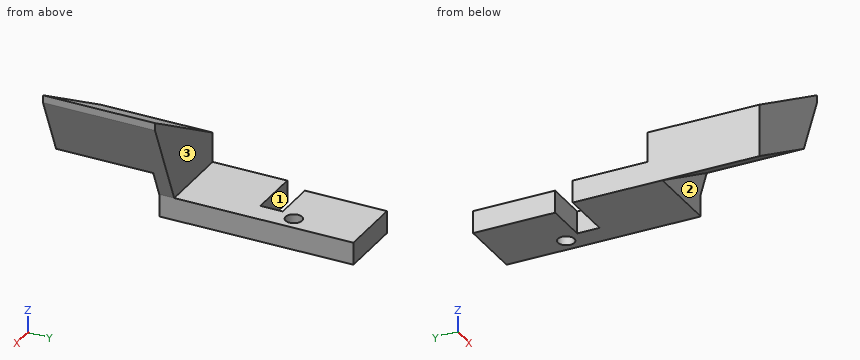
from build123d import *

# Parameters (mm, degrees)
SKETCH1_R           = 1.1
BOSS_EXTRUDE1_DEPTH = 3
SKETCH2_W           = 10
SKETCH2_H           = 25
BOSS_EXTRUDE2_DEPTH = 3
SKETCH3_W           = 5
SKETCH3_H           = 3
SKETCH3_W_2         = 10
BOSS_EXTRUDE3_DEPTH = 15
CUT_EXTRUDE1_DEPTH  = 15
CUT_EXTRUDE3_DEPTH  = 13


with BuildPart() as part:
    # Sketch1 → Boss-Extrude1 (new body)
    with BuildSketch(Plane.XY):
        Polygon((4.875, 7), (-3.875, 7), (-3.875, -4), (1.875, -4), (1.875, -7), (4.875, -7), align=None)
        with Locations((2.875, -2)):
            Circle(SKETCH1_R, mode=Mode.SUBTRACT)
    extrude(amount=BOSS_EXTRUDE1_DEPTH)

    # Sketch2 → Boss-Extrude2 (add)
    with BuildSketch(Plane.XY.offset(3)):
        with Locations((-0.125, -19.5)):
            Rectangle(SKETCH2_W, SKETCH2_H)
    extrude(amount=-BOSS_EXTRUDE2_DEPTH)

    # Sketch3 → Boss-Extrude3 (add)
    with BuildSketch(Plane(origin=(0, -32, 0), x_dir=(-1, 0, 0), z_dir=(0, -1, 0))):
        Polygon((-9.875, -11.660254038), (5.125, -3), (-4.875, -3), (-9.875, -3), align=None)
        with Locations((-7.375, -1.5)):
            Rectangle(SKETCH3_W, SKETCH3_H)
        with Locations((0.125, -1.5)):
            Rectangle(SKETCH3_W_2, SKETCH3_H)
        Polygon((5.125, -7), (-9.875, -15.660254038), (-9.875, -11.660254038), (5.125, -3), align=None)
    extrude(amount=-BOSS_EXTRUDE3_DEPTH)

    # Sketch5 → Cut-Extrude1 (cut)
    with BuildSketch(Plane(origin=(0, -17, 0), x_dir=(1, 0, 0), z_dir=(0, 1, 0))):
        Polygon((9.875, -14.660254038), (4.875, -3), (4.875, 0), (9.875, 0), align=None)
    extrude(amount=-CUT_EXTRUDE1_DEPTH, mode=Mode.SUBTRACT)

    # Sketch6 → Cut-Extrude3 (cut)
    with BuildSketch(Plane(origin=(0, -32, 0), x_dir=(-1, 0, 0), z_dir=(0, -1, 0))):
        Polygon((-6.45561312, -6.686070102), (5.125, 0), (-4.875, 0), (-4.875, -3), align=None)
    extrude(amount=-CUT_EXTRUDE3_DEPTH, mode=Mode.SUBTRACT)


solid = part.part
Input: part model. Units: mm. Frame: model coordinates. Face numbers are marked on the shaded views. A direction names the side the tool comes from. Give positions to 0.01 mm unless a question says otherwise; leave off trailing zeros. Write each loop counter-clockwise with the first axis right and the second up, starting at its lowest first coordinate (ties: lowest second). Pieces come first, ordered by that corner, then holes. Notation, with made-up numbers: M 6.25,22 L 56.25,22 A11 ccw 56.25,27 Z; hole C 49,-17.5 d10. An arc over 180 degrees is marked long. Write item = value, one per line. Start each with the question number.
1) Material intervals for line 1 along Y through (x, z) = (-3, 2.5); line 2 along X through (y, z) = (-17, 1.5) (3 decimals); line 3 along Z through (x, y) = (-0.25, 0.5), sorted ascending. Write a range as [from, to].
2) Reachability of the marked faces 1, 2 and 3 from +Z, -Z, +X, -X, +Y, -Y: full face, straight path, thin tool, end or side. Return the list, or none.
3) Cut plane B-B on x = 1.25. Return the cut outline in (y, z).
4) Cut plane D-D on x = -3. Return the cut outline in (y, z), then the cut area to 3 significant figures.
5) First-contact query: pin 1 Ø3.5 at (y, z) = (-0.5, 1.5) entering from -X (3 decimals); pin 2 Ø0.9 at (y, z) = (-3.5, 2) entering from +X (3 decimals); pin 3 Ø2 at (x, z) = (2, 2.5) entering from -Y; pin 4 Ø1.3 at (x, y) = (2.875, -2) entering from +Z. Flat tips, straight axial feed; report the tip coordinate or a pass-through.
6) Cut plane A-A on y = -2. Return the cut outline in (x, z) (3 decimals).
7) Cut plane C-C on z = 1.5. Return the cut outline in (x, y) (3 decimals).
Solved:
q1.line_1 = [-32, -7], [-4, 7]
q1.line_2 = [-5.125, 4.875]
q1.line_3 = [0, 3]
q2.face_1 = +Z, -Z, -X
q2.face_2 = -Z, +X, -Y
q2.face_3 = +Z, +X, -X, +Y
q3.outline = M -32,3.68 L -19,3.68 L -19,0 L -7,0 L -7,3 L -17,3 L -17,10.68 L -32,10.68 Z; M -4,0 L 7,0 L 7,3 L -4,3 Z
q4.outline = M -32,1.23 L -19,1.23 L -19,0 L -7,0 L -7,3 L -17,3 L -17,8.23 L -32,8.23 Z; M -4,0 L 7,0 L 7,3 L -4,3 Z
q4.area = 170 mm2
q5.pin_1 = -3.875
q5.pin_2 = 4.875
q5.pin_3 = -19
q5.pin_4 = through
q6.outline = M -3.875,0 L 1.775,0 L 1.775,3 L -3.875,3 Z; M 3.975,0 L 4.875,0 L 4.875,3 L 3.975,3 Z
q7.outline = M -5.125,-32 L -2.527,-32 L -2.527,-19 L 4.875,-19 L 4.875,7 L -3.875,7 L -3.875,-4 L 1.875,-4 L 1.875,-7 L -5.125,-7 Z; hole C 2.875,-2 d2.2
